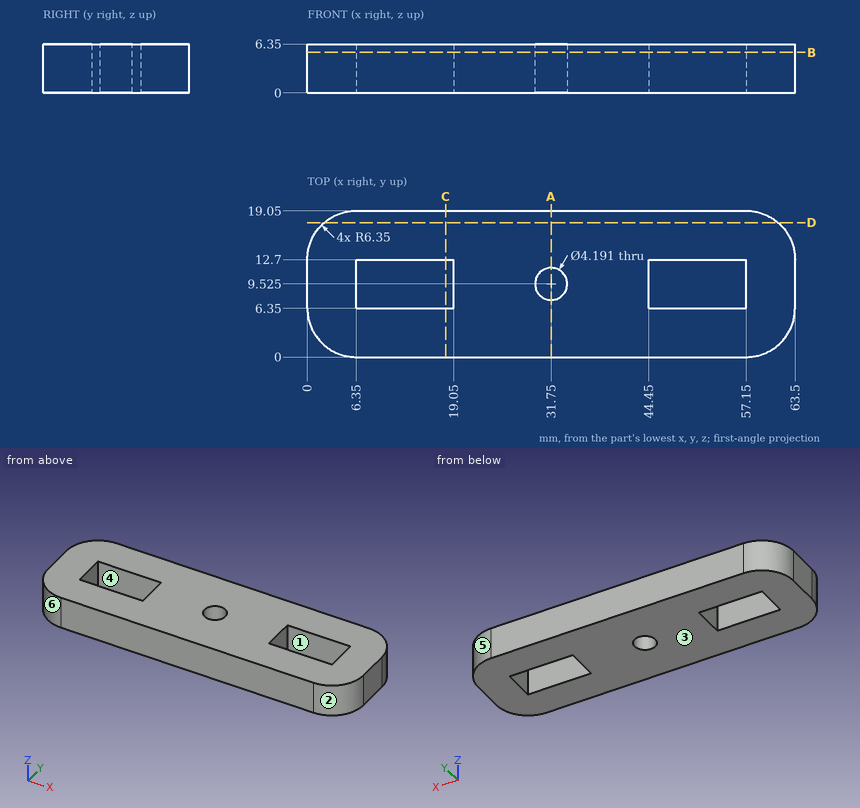
Part print with two shaded views. Sizes in mm from the minimum x, y, z corner. A direction names the side the tool comes from. Give positions to 0.01 mm unless a question says otherwise; leave off trailing zeros. Write each loop counter-clockwise with the first axis right and the second up, starting at its lowest first coordinate (ties: lowest second). Pieces come first, ordered by that corner, then holes.
1) Cut at A-A on x = 31.75. Write the cut outline in (y, z).
Resolved:
outline: (0, 0) - (7.43, 0) - (7.43, 6.35) - (0, 6.35) - close; (11.62, 0) - (19.05, 0) - (19.05, 6.35) - (11.62, 6.35) - close
2) Which spindle directions (+Z, -Z, +X, -X, +Y, -Y) get a long thin tool onto all of the face, cutting with end or side? Do the marked faces 1 and 2. Say none if no direction does.
Resolved:
face 1: +Z, -Z
face 2: +Z, -Z, +X, -Y
3) Cut at D-D on y = 17.5. Write the cut outline in (x, z).
Resolved:
outline: (2.19, 0) - (61.31, 0) - (61.31, 6.35) - (2.19, 6.35) - close
4) Cut at C-C on x = 18. Write the cut outline in (y, z), then the cut area to 3 significant figures.
Resolved:
outline: (0, 0) - (6.35, 0) - (6.35, 6.35) - (0, 6.35) - close; (12.7, 0) - (19.05, 0) - (19.05, 6.35) - (12.7, 6.35) - close
area: 80.6 mm2
5) Cut at B-B on z = 5.25. State how many separate pieces and enclosed holes the cut face has, then the cut area to 4 significant figures.
Resolved:
separate pieces: 1
enclosed holes: 3
area: 1,000 mm2
6) Probe L1, parallel to X at y = 6.5, z = 1.25; L2, parallel to Y at x = 31.75, z = 4; L3, parallel to Y at x = 54, z = 5.25. List the from-to ranges inside material, lowest first.
Resolved:
L1: x = 0 to 6.35, 19.05 to 44.45, 57.15 to 63.5
L2: y = 0 to 7.43, 11.62 to 19.05
L3: y = 0 to 6.35, 12.7 to 19.05
7) Two-plate mould, pull along X, no slides. Class the marked faces 3, 4, 5 and 6: released by +X, released by -X, zero draft, split by the parting line, or undercut.
Resolved:
face 3: zero draft
face 4: undercut
face 5: released by +X
face 6: released by -X
